The model under review builds one solid part; all positions refer to its coordinate system, in mm. A direction names the side the tool comes from. Coordinates: 2 decimals unless noted, no trailing zeros. Loops run counter-clockwise (first coordinate to the right, second up) from the corner with the lowest first, then second, coordinate; pieces in that order, holes last. Notation, with made-up numbers: M 85.25,43 L 109.25,43 A17 cw 109.25,63 Z; hole C 21,40.5 d6. An arc over 180 degrees is marked long. Write item = value, one per line. Start each with the question number.
Q1. Mouldability with a two-part tool opening along Y and no side actions: class faces 4 (the face through (-2, 16, 16)), 5 (the face through (-32, 8, 3)), 6 (the face through (-12, -6, 3)) as released by +Y, released by -Y, zero draft, split by the parting line, or undercut.
Q2. Clearance check with flat-ended pins moving along their axes: pin 1 Ø6.5 at (x, z) = (-22.5, 9.5) entering from +Y; pin 2 Ø5.5 at (x, y) = (2.5, 14) entering from +Z; pin 3 Ø12 at (x, y) = (1.5, 9.5) entering from +Z. State where each tip first meets the part, or that it passes through.
Q3. We need section D-D on x = -1. Give the boundary of the cut face in (y, z), and give its area (3 significant figures).
Q4. For faces 1 (the face through (-9, 16, 20)), 2 (the face through (9, 12, 11)), 3 (the face through (30, -5, 3)), list the 3-axis set-ups (+Z, -Z, +X, -X, +Y, -Y) from which the entire face can be reached by the end or side of a thin tool; tool diameter is ignored.
Q5. We need section C-C on y = -10. Give the boundary of the cut face in (x, z).
Q6. We need section B-B on x = -10. Give the boundary of the cut face in (y, z), and give its area (3 significant figures).
Q7. We need section A-A on z = 4.5. Give the boundary of the cut face in (x, y).
Q8. Wall thickness on probe 1 along Z at (x, y) = (10, -4.5); probe 2 along Y at (x, z) = (-19, 6.75); probe 3 along Z at (x, y) = (18.5, 25): over which ranges is each line inside the solid? List them lowest first.
from build123d import *

# Parameters (mm, degrees)
EXTRUDE_1_DEPTH     = 6
EXTRUDE_3_DEPTH     = 8
SKETCH_3_W          = 3
SKETCH_3_H          = 14
CUT_EXTRUDE_1_DEPTH = 47
SKETCH_4_W          = 50.5
SKETCH_4_H          = 7
EXTRUDE_4_DEPTH     = 20
CUT_EXTRUDE_2_REACH = 67.59
SKETCH_5_W          = 13.5
SKETCH_5_H          = 6
SKETCH_5_W_2        = 15
SKETCH_5_H_2        = 10


with BuildPart() as part:
    # Эскиз1 → Бобышка-Вытянуть1 (new body)
    with BuildSketch(Plane.XY):
        Polygon((-35, 8), (-35, -30), (25, -30), (25, -5), (35, -5), (35, 30), (-15.5, 30), (-15.5, 12), (-29, 12), (-29, 8), align=None)
    extrude(amount=EXTRUDE_1_DEPTH)

    # Эскиз2 → Бобышка-Вытянуть3 (add)
    with BuildSketch(Plane.XZ.offset(30)):
        Polygon((-35, 6), (-35, 9), (-15.5, 14), (-15.5, 6), align=None)
    extrude(amount=-EXTRUDE_3_DEPTH)

    # Эскиз3 → Вырез-Вытянуть1 (cut)
    with BuildSketch(Plane.ZY.offset(35)):
        with Locations((1.5, -6)):
            Rectangle(SKETCH_3_W, SKETCH_3_H)
    extrude(amount=-CUT_EXTRUDE_1_DEPTH, mode=Mode.SUBTRACT)

    # Эскиз4 → Бобышка-Вытянуть4 (add)
    with BuildSketch(Plane.XY.offset(6)):
        with Locations((9.75, 15.5)):
            Rectangle(SKETCH_4_W, SKETCH_4_H)
    extrude(amount=EXTRUDE_4_DEPTH)

    # Эскиз5 → Вырез-Вытянуть2 (cut, up to next)
    with BuildSketch(Plane(origin=(0, 19, 0), x_dir=(1, 0, 0), z_dir=(0, 1, 0)), mode=Mode.PRIVATE) as cut_extrude_2_sk1:
        Polygon((-2, -26), (10, -26), (10, -13), (-2, -13), (-2, -20), align=None)
    cut_extrude_2_tool1 = extrude(cut_extrude_2_sk1.sketch, amount=-CUT_EXTRUDE_2_REACH, mode=Mode.PRIVATE) & part.part
    # Эскиз5 → Вырез-Вытянуть2 (cut, up to next)
    with BuildSketch(Plane(origin=(0, 19, 0), x_dir=(1, 0, 0), z_dir=(0, 1, 0)), mode=Mode.PRIVATE) as cut_extrude_2_sk2:
        with Locations((-8.75, -23)):
            Rectangle(SKETCH_5_W, SKETCH_5_H)
    cut_extrude_2_tool2 = extrude(cut_extrude_2_sk2.sketch, amount=-CUT_EXTRUDE_2_REACH, mode=Mode.PRIVATE) & part.part
    # Эскиз5 → Вырез-Вытянуть2 (cut, up to next)
    with BuildSketch(Plane(origin=(0, 19, 0), x_dir=(1, 0, 0), z_dir=(0, 1, 0)), mode=Mode.PRIVATE) as cut_extrude_2_sk3:
        with Locations((27.5, -21)):
            Rectangle(SKETCH_5_W_2, SKETCH_5_H_2)
    cut_extrude_2_tool3 = extrude(cut_extrude_2_sk3.sketch, amount=-CUT_EXTRUDE_2_REACH, mode=Mode.PRIVATE) & part.part
    add(cut_extrude_2_tool1.solids().sort_by_distance((4, 19, 19.5))[0], mode=Mode.SUBTRACT)
    add(cut_extrude_2_tool2.solids().sort_by_distance((-8.75, 19, 23))[0], mode=Mode.SUBTRACT)
    add(cut_extrude_2_tool3.solids().sort_by_distance((27.5, 19, 21))[0], mode=Mode.SUBTRACT)


solid = part.part
Returned:
q1.face_4 = zero draft
q1.face_5 = released by +Y
q1.face_6 = undercut
q2.pin_1 = -22
q2.pin_2 = 13
q2.pin_3 = 20
q3.outline = M -30,0 L -13,0 L -13,3 L 1,3 L 1,0 L 30,0 L 30,6 L 19,6 L 19,13 L 12,13 L 12,6 L -30,6 Z
q3.area = 367 mm^2
q4.face_1 = +Z, -X, +Y, -Y
q4.face_2 = +Z, +X, -X, -Y
q4.face_3 = +Z, -Z, +X, -Y
q5.outline = M -35,3 L 12,3 L 12,0 L 25,0 L 25,6 L -35,6 Z
q6.outline = M -30,0 L -13,0 L -13,3 L 1,3 L 1,0 L 30,0 L 30,6 L 19,6 L 19,20 L 12,20 L 12,6 L -30,6 Z
q6.area = 416 mm^2
q7.outline = M -35,-30 L 25,-30 L 25,-5 L 35,-5 L 35,30 L -15.5,30 L -15.5,12 L -29,12 L -29,8 L -35,8 Z
q8.probe_1 = 3 to 6
q8.probe_2 = -30 to -22
q8.probe_3 = 0 to 6
